Autodesk Inventor part; units mm, degrees
ref_plane "YZ Plane" through (0, 0, 0) normal (1, 0, 0) x (0, 1, 0)
ref_plane "XZ Plane" through (0, 0, 0) normal (0, 1, 0) x (-1, 0, 0)
ref_plane "XY Plane" through (0, 0, 0) normal (0, 0, 1) x (1, 0, 0)
sketch "Sketch1" plane through (0, 0, 0) normal (1, 0, 0) x (0, 1, 0)
  circle A0 centre (27.94, -44.6106) radius 6.985 construction
  circle A1 centre (50.8, -18.5683) radius 6.35 construction
  line L0 (63.5, 0) -> (50.8, 0) construction
  line L1 (50.8, 0) -> (50.8, -12.7) construction
  line L2 (50.8, -12.7) -> (63.5, -12.7) construction
  line L3 (63.5, -12.7) -> (63.5, 0) construction
  circle A2 centre (50.8, -70.0106) radius 6.35 construction
  line L4 (27.94, -31.779) -> (39.0525, -38.1948) construction
  line L5 (39.0525, -38.1948) -> (39.0525, -51.0264) construction
  line L6 (39.0525, -51.0264) -> (27.94, -57.4422) construction
  line L7 (27.94, -57.4422) -> (16.8275, -51.0264) construction
  line L8 (16.8275, -51.0264) -> (16.8275, -38.1948) construction
  line L9 (63.5, 0) -> (0, 0)
  line L10 (0, -88.9) -> (63.5, -88.9)
  line L11 (63.5, -88.9) -> (63.5, 0)
  line L12 (0, -44.45) -> (27.94, -44.45) construction
  line L13 (0, -44.45) -> (27.94, -44.45) construction
  line L14 (27.94, -31.779) -> (16.8275, -38.1948) construction
  line L15 (0, -44.45) -> (63.5, -44.45) construction
  line L16 (0, -44.45) -> (0, -60.325) construction
  line L17 (0, -44.45) -> (15.875, -44.45) construction
  line L18 (0, -60.325) -> (-12.7, -60.325)
  line L19 (-12.7, -60.325) -> (-12.7, -73.025)
  line L20 (-12.7, -73.025) -> (0, -73.025)
  line L21 (0, -44.45) -> (0, -28.575) construction
  line L22 (0, -28.575) -> (-12.7, -28.575)
  line L23 (-12.7, -28.575) -> (-12.7, -15.875)
  line L24 (-12.7, -15.875) -> (0, -15.875)
  line L25 (0, 0) -> (0, -15.875)
  line L26 (0, -28.575) -> (0, -60.325)
  line L27 (0, -73.025) -> (0, -88.9)
  point P0 (0, 0)
  point P1 (0, -12.8606)
  dimension "d13" = 88.9
  dimension "d14" = 63.5
  dimension "d15" = 15.875
  dimension "d16" = 90
  dimension "d17" = 12.7
  dimension "d18" = 12.7
extrude "Extrusion2" add sketch "Sketch1" along normal blind 12.7
sketch "Sketch2" plane through (12.7, 0, 0) normal (1, 0, 0) x (0, 0, -1)
  circle A0 centre (45.5875, 27.94) radius 6.985
  circle A1 centre (19.5452, 50.8) radius 6.35
  circle A2 centre (70.9875, 50.8) radius 6.35
  line L0 (32.7559, 27.94) -> (39.1717, 39.0525) construction
  line L1 (39.1717, 39.0525) -> (52.0033, 39.0525) construction
  line L2 (52.0033, 39.0525) -> (58.4191, 27.94) construction
  line L3 (58.4191, 27.94) -> (52.0033, 16.8275) construction
  line L4 (52.0033, 16.8275) -> (39.1717, 16.8275) construction
  line L5 (45.4269, 0) -> (45.4269, 27.94) construction
  line L6 (32.7559, 27.94) -> (39.1717, 16.8275) construction
  line L7 (88.9, 0) -> (88.9, 63.5) construction
  line L8 (0, 0) -> (88.9, 0) construction
  line L9 (28.575, 0) -> (60.325, 0) construction
  line L10 (44.45, 0) -> (44.45, 63.5) construction
  line L11 (88.9, 63.5) -> (0, 63.5) construction
  line L12 (44.45, 0) -> (44.45, 27.94) construction
  line L13 (44.45, 0) -> (72.39, 0) construction
  dimension "d25" = 27.94
  dimension "d26" = 90
extrude "Extrusion3" cut sketch "Sketch2" against normal blind 6.35
sketch "Sketch3" plane through (12.7, 0, 0) normal (1, 0, 0) x (0, 0, -1)
  line L0 (0, 25.4) -> (6.35, 25.4)
  line L1 (6.35, 25.4) -> (6.35, 38.1)
  line L2 (6.35, 38.1) -> (0, 38.1)
  line L3 (0, 63.5) -> (0, 0)
  line L4 (0, 38.1) -> (0, 25.4)
  line L5 (88.9, 63.5) -> (0, 63.5) construction
  line L6 (44.45, 63.5) -> (44.45, 0) construction
  line L7 (28.575, 0) -> (60.325, 0) construction
  line L8 (88.9, 25.4) -> (82.55, 25.4)
  line L9 (82.55, 25.4) -> (82.55, 38.1)
  line L10 (82.55, 38.1) -> (88.9, 38.1)
  line L11 (88.9, 38.1) -> (88.9, 25.4)
  point P0 (0, 31.75)
  point P1 (88.9, 31.75)
  dimension "d28" = 12.7
extrude "Extrusion4" cut sketch "Sketch3" against normal through all
sketch "Sketch4" plane through (12.7, 0, 0) normal (1, 0, 0) x (0, 0, -1)
  line L0 (28.575, 0) -> (60.325, 0) construction
  line L1 (44.45, 0) -> (44.45, 63.5) construction
  line L2 (88.9, 63.5) -> (0, 63.5) construction
  line L3 (44.45, 63.5) -> (44.45, 69.85) construction
  line L4 (44.45, 63.5) -> (50.8, 63.5) construction
  line L5 (38.1, 76.2) -> (50.8, 76.2)
  line L6 (50.8, 76.2) -> (50.8, 63.5)
  line L7 (50.8, 63.5) -> (38.1, 63.5)
  line L8 (38.1, 63.5) -> (38.1, 76.2)
  line L9 (38.1, 76.2) -> (50.8, 63.5) construction
  line L10 (50.8, 76.2) -> (38.1, 63.5) construction
  point P0 (0, 0)
  dimension "d31" = 6.35
  dimension "d32" = 90
  dimension "d33" = 12.7
  dimension "d34" = 12.7
extrude "Extrusion5" add sketch "Sketch4" against normal blind 12.7
sketch "Sketch5" plane through (12.7, 0, 0) normal (1, 0, 0) x (0, 0, -1)
  line L0 (73.025, 0) -> (88.9, 0) construction
  line L1 (88.9, 0) -> (88.9, 19.05) construction
  line L2 (88.9, 0) -> (107.95, 0) construction
  line L3 (88.9, 19.05) -> (69.85, 19.05) construction
  circle A0 centre (69.85, 19.05) radius 9.525
  point P0 (0, 0)
  dimension "d37" = 19.05
  dimension "d38" = 90
  dimension "d39" = 19.05
  dimension "d40" = 90
  dimension "d41" = 19.05
extrude "Extrusion6" cut sketch "Sketch5" against normal through all
properties part number "Far End Cap" material "PVC-Piping"
The listing builds one solid part. Answer for the finished solid, in the listing's coordinates (mm). A direction names the side the tool comes from. Round coordinates to 2 decimals unless told otherwise and drop trailing zeros. Loops run counter-clockwise (first coordinate to the right, second up) from the corner with the lowest first, then second, coordinate; pieces in that order, holes last.
Q1. Find the intervals of material crossed by line 1 (Z direction, x = 7.5, y = -4.5) (3 decimals); line 2 (X direction, y = 54.5, z = -67); line 3 (Z direction, x = 4.5, y = 25.5), in increasing order.
Q2. Section B-B, the plane z = -62.5 is taken. Determine the outline of the cut face in (x, y).
Q3. For a pull along Z with two mould halves and no side action, classify faces 1 (the face through (9.57, 25.26, -52.04)), 2 (the face through (6, -6, -73.025)), 3 (the face through (6, -6, -28.575)), 4 (the face through (6, 13, 0)) as released by +Z, released by -Z, zero draft, split by the parting line, or undercut.
Q4. Given pin 1 Ø6 at (x, z) = (8, -52) entering from -Y; pin 2 Ø4 at (x, y) = (6, 68) entering from +Z; pin 3 Ø7 at (x, z) = (7, -3) entering from +Y, each flat-ended and moving along its own axis, determine where each tip first touches the part or whether it passes through.
Q5. Which of the six approach directions +Z, -Z, +X, -X, +Y, -Y give full straight-line access (tool end or side, diameter ignored) to faces 5 (the face through (6, 25.4, -3)), 6 (the face through (6, -6, -15.875)), 7 (the face through (6, 32, -82.55))?
Q6. Section A-A, the plane y = -4.5 is taken. Determine the outline of the cut face in (x, z) (3 decimals), then the cut area to 3 significant figures.
Q7. Section D-D, the plane y = 50.8 is taken. Determine the outline of the cut face in (x, z), then the cut area to 3 significant figures.
Q8. Section C-C, the plane x = 10 is taken. Count the separate pieces of the cut face and the enclosed holes in it, then the cut area to 3 significant figures.
Completed:
1. line 1: z = -73.025 to -60.325, -28.575 to -15.875
1. line 2: x = 0 to 6.35
1. line 3: z = -82.55 to -76.86, -62.84 to -6.35
2. outline: (0, -12.7) - (12.7, -12.7) - (12.7, 12.99) - (0, 12.99) - close; (0, 25.11) - (12.7, 25.11) - (12.7, 63.5) - (0, 63.5) - close
3. face 1: undercut
3. face 2: released by -Z
3. face 3: undercut
3. face 4: released by +Z
4. pin 1: stops at y = 0
4. pin 2: stops at z = -38.1
4. pin 3: stops at y = 63.5
5. face 5: +Z, +X, -X
5. face 6: +Z, +X, -X, -Y
5. face 7: -Z, +X, -X
6. outline: (0, -73.025) - (12.7, -73.025) - (12.7, -60.325) - (0, -60.325) - close; (0, -28.575) - (12.7, -28.575) - (12.7, -15.875) - (0, -15.875) - close
6. area: 323 mm2
7. outline: (0, -88.9) - (12.7, -88.9) - (12.7, -77.34) - (6.35, -77.34) - (6.35, -64.64) - (12.7, -64.64) - (12.7, -25.9) - (6.35, -25.9) - (6.35, -13.2) - (12.7, -13.2) - (12.7, 0) - (0, 0) - close
7. area: 968 mm2
8. separate pieces: 1
8. enclosed holes: 4
8. area: 5,280 mm2
